from build123d import *

# Parameters (mm, degrees)
SKETCH1_W                   = 19.05
SKETCH1_H                   = 34.925
BOSS_EXTRUDE1_DEPTH         = 4.7625
BOSS_EXTRUDE2_DEPTH         = 9.525
BOSS_EXTRUDE3_DEPTH         = 9.525
F_1_4_0_25_DIAMETER_HOLE1_D = 6.35
FILLET1_R                   = 6.35


with BuildPart() as part:
    # Sketch1 → Boss-Extrude1 (new, symmetric)
    with BuildSketch(Plane.XY):
        Rectangle(SKETCH1_W, SKETCH1_H)
    extrude(amount=BOSS_EXTRUDE1_DEPTH, both=True)



with BuildPart() as body_2:
    # Sketch2 → Boss-Extrude2 (new body)
    with BuildSketch(Plane.XY.offset(4.7625)):
        Polygon((9.525, 17.4625), (18.56425515, 51.197459483), (0.163368159, 56.127962292), (-8.875886991, 22.393002809), align=None)
    extrude(amount=-BOSS_EXTRUDE2_DEPTH)


with BuildPart() as part_1:
    add(part.part)

    add(body_2.part)  # Boss-Extrude3 merges body 2
    # Sketch3 → Boss-Extrude3 (add)
    with BuildSketch(Plane.XY.offset(4.7625)):
        with BuildLine():
            Line((-8.875886991, 22.393002809), (9.525, 17.4625))
            Line((9.525, 17.4625), (-9.525, 17.4625))
            ThreePointArc((-9.525, 17.4625), (-9.362024609, 19.949023962), (-8.875886991, 22.393002809))
        make_face()
    extrude(amount=-BOSS_EXTRUDE3_DEPTH)

    # 1/4 (0.25) Diameter Hole1 (through all)
    with Locations(Plane.XY.offset(4.7625)):
        with Locations((0.038567729, -0.344238019), (0.081487695, 18.705761981), (4.970520592, 37.117710746)):
            Hole(F_1_4_0_25_DIAMETER_HOLE1_D / 2)

    # Fillet1
    fillet1_edges = [part_1.edges().sort_by_distance(p)[0] for p in [
        (18.56425515, 51.197459483, 0),
        (0.163368159, 56.127962292, 0),
        (9.525, -17.4625, 0),
        (-9.525, -17.4625, 0),
        (9.525, 17.4625, 0),
    ]]
    fillet(fillet1_edges, radius=FILLET1_R)


solid = part_1.part
The model under review builds one solid part; all positions refer to its coordinate system, in mm. A direction names the side the tool comes from. Give positions to 0.01 mm unless a question says otherwise; leave off trailing zeros. Write each loop counter-clockwise with the first axis right and the second up, starting at its lowest first coordinate (ties: lowest second). Pieces come first, ordered by that corner, then holes.
1. Add section B-B, the plane z = -0.75. Count the separate pieces of the cut face and the enclosed holes in it, plus the area to 3 significant figures.
2. Wall thickness on L1, parallel to Y at x = 0.25, z = -1.25; L2, parallel to Y at x = 1.25, z = 4.25; L3, parallel to X at y = -0.5, z = -1.5 (3 decimals): over which ranges is each line inside the solid? List them lowest first.
3. Draft analysis for pull direction X (two halves, no side actions). For faces 1 (the cylindrical face through (-2.99, 0.61, -0.07)), 2 (the cylindrical face through (1.418, 53.815, -0.067)), 3 (the flat face through (13.28, 31.48, 0.07)), state which applies: +X half, -X half, draft (parallel to the pull), parting line (faces both ways), or undercut.
4. Add section A-A, the plane x = 0. Write out the cut boundary in (y, z).
5. For P1, Ø4, axis at y = -5.5, z = 1.5, coming from the +X side (3 decimals); P2, Ø4, axis at x = 0.08, y = 18.71, coming from the -Z side; P3, Ø2, axis at x = 5, z = 1, coming from the -Y side, all flat-tipped, find the tip position at first contact; note any pin that passes through.
6. Add section C-C, the plane x = 4.25. Write out the cut boundary in (y, z), plus the area to 3 significant figures.
7. Add section D-D, the plane y = 8. Write out the cut boundary in (x, z) (1 decimal).
8. Tool access review of faces 4 (the flat face through (0, -17.462, 0)), 5 (the flat face through (9.525, 3, 0)): name each direction out of +Z, -Z, +X, -X, +Y, -Y from which nothing blocks a thin tool from reaching the whole face with its end or side.
Worked answers:
1. separate pieces: 1
1. enclosed holes: 3
1. area: 1,250 mm2
2. L1: y = -17.46 to -3.51, 2.82 to 15.54, 21.88 to 52.93
2. L2: y = -17.46 to -3.28, 2.59 to 15.75, 21.66 to 53.71
2. L3: x = -9.525 to -3.133, 3.21 to 9.525
3. face 1: undercut
3. face 2: parting line
3. face 3: +X half
4. outline: (-17.46, -4.76) - (-3.52, -4.76) - (-3.52, 4.76) - (-17.46, 4.76) - close; (2.83, -4.76) - (15.53, -4.76) - (15.53, 4.76) - (2.83, 4.76) - close; (21.88, -4.76) - (52.67, -4.76) - (52.67, 4.76) - (21.88, 4.76) - close
5. P1: stops at x = 9.525
5. P2: passes through
5. P3: stops at y = -17.41
6. outline: (-17.37, -4.76) - (34.03, -4.76) - (34.03, 4.76) - (-17.37, 4.76) - close; (40.21, -4.76) - (54.69, -4.76) - (54.69, 4.76) - (40.21, 4.76) - close
6. area: 627 mm2
7. outline: (-9.5, -4.8) - (9.5, -4.8) - (9.5, 4.8) - (-9.5, 4.8) - close
8. face 4: +Z, -Z, +X, -X, -Y
8. face 5: +Z, -Z, +X, -Y
